Verification items for the finished model (mm, model axes). Face numbers are marked on the shaded views. A direction names the side the tool comes from. Give positions to 0.01 mm unless a question says otherwise; leave off trailing zeros. Write each loop counter-clockwise with the first axis right and the second up, starting at its lowest first coordinate (ties: lowest second). Pieces come first, ordered by that corner, then holes. Notation, with made-up numbers: (6, -33.5) -> (54, -33.5) arc R28 cw to (54, -12.5) -> close; hole circle Ø7 at (39, -23). An arc over 180 degrees is marked (long way). Use one line per item in the form item = value. Start each with the question number.
(1) Section check C-C, the plane y = 9. Record the cut outline in (x, z), plus the area to 3 significant figures.
(2) Release check for a two-part mould opening along X. For the marked faces 1, 2, 3 and 4 record: pulls with the +X half, pulls with the -X half, needs draft (parallel to the pull), parting line crosses it, or undercut.
(3) Section check B-B, the plane z = -33. Record the cut outline in (x, y), plus the area to 3 significant figures.
(4) Section check A-A, the plane x = 0. Record the cut outline in (y, z), plus the area to 3 significant figures.
(5) Depth check by flat-ended pin: pin 1 Ø7.5 at (y, z) = (-16, -21.5) entering from -X; pin 2 Ø5 at (x, y) = (-21.5, -64.5) entering from -Z; pin 3 Ø8.5 at (x, z) = (99, 10) entering from -Y. Enter the tip coordinate at first touch or a pass-through.
(6) Section check D-D, the plane z = -72. Record the cut outline in (x, y), plus the area to 3 significant figures.
(7) Scan lines: L1, parallel to Z at x = -68.5, y = 20; L2, parallel to Y at x = 57, z = -58.5; L3, parallel to Y at x = 73.5, z = -29. Record each from-to range of solid material in increasing order.
(8) Set-up check for the marked faces 5, 6 and 7: record each of +Z, -Z, +X, -X, +Y, -Y from which the full face is reachable in a straight line by a thin tool's end or side.
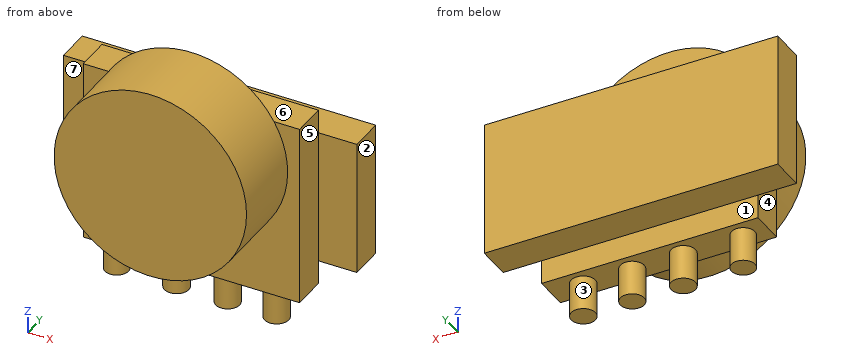
from build123d import *

# Parameters (mm, degrees)
F0_W     = 159.117624
F0_H     = 135.05447
F1_DEPTH = 25.4
F2_R     = 70.761251
F3_DEPTH = 55.626
F4_R     = 8.644359
F4_R_2   = 9.020495
F4_R_3   = 8.787981
F4_R_4   = 8.934689
F5_DEPTH = 25.4
F6_W     = 215.815008
F6_H     = 99.81057
F7_DEPTH = 25.4


with BuildPart() as f1:
    # F0 (on Front) → F1 (new body)
    with BuildSketch(Plane.XZ):
        Rectangle(F0_W, F0_H)
    extrude(amount=F1_DEPTH)

    # F2 (on face) → F3 (join)
    with BuildSketch(Plane.XZ.offset(25.4)):
        with Locations((0, 31.224668)):
            Circle(F2_R)
    extrude(amount=F3_DEPTH)

    # F4 (on face) → F5 (join)
    with BuildSketch(Plane(origin=(0, 0, -67.527235), x_dir=(1, 0, 0), z_dir=(0, 0, -1))):
        with Locations((-61.597422, 13.11885)):
            Circle(F4_R)
        with Locations((-17.532768, 13.11885)):
            Circle(F4_R_2)
        with Locations((20.015284, 13.11885)):
            Circle(F4_R_3)
        with Locations((56.011762, 13.11885)):
            Circle(F4_R_4)
    extrude(amount=F5_DEPTH)

    # F6 (on face) → F7 (join)
    with BuildSketch(Plane(origin=(0, 0, 0), x_dir=(-1, 0, 0), z_dir=(0, 1, 0))):
        Rectangle(F6_W, F6_H)
    extrude(amount=F7_DEPTH)


solid = f1.part
Completed:
q1.outline = (-107.91, -49.91) -> (107.91, -49.91) -> (107.91, 49.91) -> (-107.91, 49.91) -> close
q1.area = 21,500 mm²
q2.face_1 = needs draft
q2.face_2 = pulls with the +X half
q2.face_3 = undercut
q2.face_4 = pulls with the -X half
q3.outline = (-107.91, 0) -> (-79.56, 0) -> (-79.56, -25.4) -> (-29.7, -25.4) -> (-29.7, -81.03) -> (29.7, -81.03) -> (29.7, -25.4) -> (79.56, -25.4) -> (79.56, 0) -> (107.91, 0) -> (107.91, 25.4) -> (-107.91, 25.4) -> close
q3.area = 12,800 mm²
q4.outline = (-81.03, -39.54) -> (-25.4, -39.54) -> (-25.4, -67.53) -> (0, -67.53) -> (0, -49.91) -> (25.4, -49.91) -> (25.4, 49.91) -> (0, 49.91) -> (0, 67.53) -> (-25.4, 67.53) -> (-25.4, 101.99) -> (-81.03, 101.99) -> close
q4.area = 13,800 mm²
q5.pin_1 = -79.56
q5.pin_2 = -36.94
q5.pin_3 = 0
q6.outline = circle Ø17.29 at (-61.6, -13.12); circle Ø18.04 at (-17.53, -13.12); circle Ø17.58 at (20.02, -13.12); circle Ø17.87 at (56.01, -13.12)
q6.area = 984 mm²
q7.L1 = -49.91 to 49.91
q7.L2 = -25.4 to 0
q7.L3 = -25.4 to 25.4
q8.face_5 = +Z, -Z, +X, -Y
q8.face_6 = +Z, +X, -X, +Y
q8.face_7 = +Z, -Z, -X, -Y
